Input: part model. Units: mm. Frame: model coordinates. Face numbers are marked on the shaded views. A direction names the side the tool comes from. Round coordinates to 2 decimals unless told otherwise and drop trailing zeros. Loops run counter-clockwise (first coordinate to the right, second up) from the corner with the lowest first, then second, coordinate; pieces in that order, holes last. Notation, with made-up numbers: M 35.5,74 L 39.5,74 A35 cw 39.5,113 Z; hole C -20.5,-19 d5. An arc over 180 degrees is marked long. Return JSON: item names as keys, results as strings. Group by question number.
1) Material intervals for line 1 (Y direction, x = 0, z = 58.5); line 2 (Z direction, x = 58, y = -48); line 3 (Z direction, x = -56, y = 21), sorted ascending. Write a range as from..to.
2) Section B-B (z = 3). Output: boundary loops of the cut face in (x, y), plus the area to 3 significant figures.
3) Section A-A (z = 87.5). Output: boundary loops of the cut face in (x, y).
4) Access query for the marked faces 1 and 2. Directions: +Z, -Z, +X, -X, +Y, -Y. A direction counts if a zero-diameter tool reaches every point of the face in a straight line with its end or side. Return the directions, or none.
5) Contact query for flat-ended pins moving along their axis: P1, Ø23.5, axis at x = -1.5, y = 0.5, coming from the +Z side; P2, Ø12, axis at y = 11, z = 75.5, coming from the +X side; P3, Ø8, axis at y = 3.5, z = 109, coming from the -X side; P4, Ø10, axis at x = -5.5, z = 18.5, coming from the -Y side. Output: stop coordinate, or through.
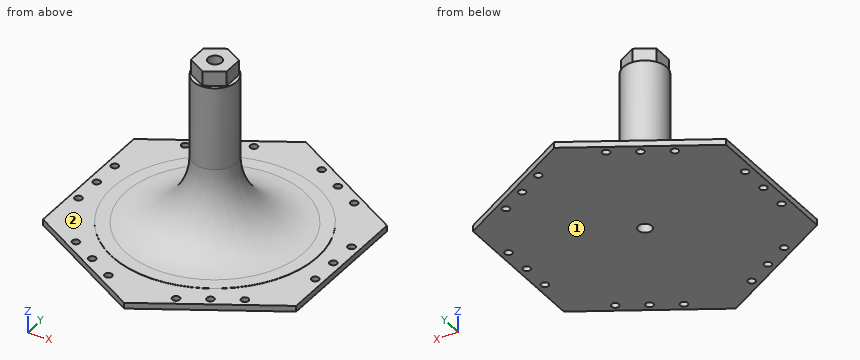
from build123d import *

# Parameters (mm, degrees)
SKETCH001_R        = 4.7
PAD_DEPTH          = 4
SKETCH002_R        = 4.7
PAD001_DEPTH       = 10
SKETCH003_R        = 2.55
POCKET_DEPTH       = 5
POLARPATTERN_COUNT = 6


with BuildPart() as part:
    # Sketch → Revolution (revolve)
    with BuildSketch(Plane.XZ):
        with BuildLine():
            Line((14.8, 46.4), (14.8, 103))
            Line((14.8, 103), (4.7, 103))
            Line((4.7, 103), (4.7, 0))
            Line((4.7, 0), (70, 0))
            Line((70, 0), (70, 0.2))
            Line((70, 0.2), (61, 0.2))
            ThreePointArc((14.8, 46.4), (28.331667, 13.731667), (61, 0.2))
        make_face()
    revolve(axis=Axis((0, 0, 0), (0, 0, 1)))

    # Sketch001 (on Face4 of Revolution) → Pad (new body)
    with BuildSketch(Plane(origin=(0, 0, 0), x_dir=(1, 0, 0), z_dir=(0, 0, -1))):
        Polygon((0, 100), (-86.60254, 50), (-86.60254, -50), (0, -100), (86.60254, -50), (86.60254, 50), align=None)
        Circle(SKETCH001_R, mode=Mode.SUBTRACT)
    extrude(amount=PAD_DEPTH)

    # Sketch002 (on Face3 of Pad) → Pad001 (join)
    with BuildSketch(Plane(origin=(0, 0, 103), x_dir=(-1, 0, 0), z_dir=(0, 0, 1))):
        Polygon((0, 14), (-12.124356, 7), (-12.124356, -7), (0, -14), (12.124356, -7), (12.124356, 7), align=None)
        Circle(SKETCH002_R, mode=Mode.SUBTRACT)
    extrude(amount=PAD001_DEPTH)

    # Sketch003 (on Face28 of Pad001) → Pocket (cut)
    with BuildSketch(Plane(origin=(0, 0, -4), x_dir=(1, 0, 0), z_dir=(0, 0, -1))):
        with Locations((-57.807196, 60.125)):
            Circle(SKETCH003_R)
        with Locations((-40.486688, 70.125)):
            Circle(SKETCH003_R)
        with Locations((-23.16618, 80.125)):
            Circle(SKETCH003_R)
    pocket = extrude(amount=-POCKET_DEPTH, mode=Mode.SUBTRACT)

    # PolarPattern: Pocket ×6 about axis
    polarpattern_axis = Axis((0, 0, -4), (0, 0, -1))
    for i in range(1, POLARPATTERN_COUNT):
        add(pocket.rotate(polarpattern_axis, i * 360 / POLARPATTERN_COUNT), mode=Mode.SUBTRACT)


solid = part.part
Returned:
{
 "1": {"line 1": "y = -14.8..-4.7, 4.7..14.8", "line 2": "z = -4..0", "line 3": "z = -4..0.22"},
 "2": {"outline": "C 0,0 d90.32; hole C 0,0 d9.4", "area": "6,340 mm^2"},
 "3": {"outline": "C 0,0 d29.6; hole C 0,0 d9.4"},
 "4": {"face 1": "-Z, +X, -X, +Y, -Y", "face 2": "+Z"},
 "5": {"P1": "stops at z = 113", "P2": "stops at x = 13.93", "P3": "stops at x = -12.12", "P4": "stops at y = -28.11"}
}
